```python
from build123d import *

# Parameters (mm, degrees)
CUT_EXTRUDE1_REACH             = 24.669
SKETCH2_R                      = 0.9525
CUT_EXTRUDE1_DIRECTION_2_REACH = 24.669


with BuildPart() as part:
    # Sketch3 → Revolve1 (revolve)
    with BuildSketch(Plane(origin=(0, 0, 0), x_dir=(0, 0, -1), z_dir=(1, 0, 0)), mode=Mode.PRIVATE) as revolve1_sk:
        with BuildLine():
            Line((-4.7625, 7.1247), (-4.7625, 9.50595))
            ThreePointArc((-4.7625, 9.50595), (-0.2272742, 11.825581937), (3.112721606, 15.6718))
            Line((3.112721606, 15.6718), (4.7625, 14.7193))
            Line((4.7625, 14.7193), (2.305035487, 10.462846606))
            ThreePointArc((2.305035487, 10.462846606), (2.305035487, 9.824915535), (2.8575, 9.50595))
            Line((2.8575, 9.50595), (4.28625, 9.50595))
            Line((4.28625, 9.50595), (4.28625, 7.1247))
            Line((4.28625, 7.1247), (-4.7625, 7.1247))
        make_face()
    revolve(revolve1_sk.sketch.rotate(Axis((0, 0, 4.7625), (0, 0, -1)), 180), axis=Axis((0, 0, 4.7625), (0, 0, -1)))

    # Sketch2 → Cut-Extrude1 (cut, up to next)
    with BuildSketch(Plane(origin=(0, 0, 0), x_dir=(0, 0, -1), z_dir=(1, 0, 0)), mode=Mode.PRIVATE) as cut_extrude1_sk1:
        with Locations((4.7625, 0)):
            Circle(SKETCH2_R)
    cut_extrude1_tool1 = extrude(cut_extrude1_sk1.sketch, amount=-CUT_EXTRUDE1_REACH, mode=Mode.PRIVATE) & part.part
    add(cut_extrude1_tool1.solids().sort_by_distance((0, 0, -4.7625))[0], mode=Mode.SUBTRACT)

    # Sketch2 → Cut-Extrude1 direction 2 (cut, up to next)
    with BuildSketch(Plane(origin=(0, 0, 0), x_dir=(0, 0, -1), z_dir=(1, 0, 0)), mode=Mode.PRIVATE) as cut_extrude1_direction_2_sk1:
        with Locations((4.7625, 0)):
            Circle(SKETCH2_R)
    cut_extrude1_direction_2_tool1 = extrude(cut_extrude1_direction_2_sk1.sketch, amount=CUT_EXTRUDE1_DIRECTION_2_REACH, mode=Mode.PRIVATE) & part.part
    add(cut_extrude1_direction_2_tool1.solids().sort_by_distance((0, 0, -4.7625))[0], mode=Mode.SUBTRACT)


solid = part.part
```
Input: part model. Units: mm. Frame: model coordinates. A direction names the side the tool comes from. Round coordinates to 2 decimals unless told otherwise and drop trailing zeros. Order: outer loops, then holes, each group sorted by start corner. A loop starts at its lowest first (then second) coordinate and runs counter-clockwise, first axis right, second up. Notation, with made-up numbers: (67, 83.5) - (87, 83.5) arc R13 cw to (87, 93.5) - close; hole circle Ø9 at (34.5, 19). An arc over 180 degrees is marked (long way). Answer in a Markdown table with one row per item.
Item 1: Section query C-C (z = 1.75). Return the cut outline in (x, y), then the cut area to 3 significant figures.
Model answer:
| item | result |
|---|---|
| outline | circle Ø21.59 at (0, 0); hole circle Ø14.25 at (0, 0) |
| area | 207 mm² |
Item 2: Mould query, pull axis X, two halves, no side actions, for faces 3 (the conical face through (-3.205, -10.177, -2.424)), 4 (the flat face through (-6.4, 3.5, 4.762)). Classes: released by +X, released by -X, zero draft, split by the parting line, or undercut.
Model answer:
| item | result |
|---|---|
| face 3 | undercut |
| face 4 | zero draft |
Item 3: Section query B-B (y = 0). Return the cut outline in (x, z), then the cut area to 3 significant figures.
Model answer:
| item | result |
|---|---|
| outline | (-15.67, -3.11) - (-14.72, -4.76) - (-10.46, -2.31) arc R0.64 cw to (-9.51, -2.86) - (-9.51, -3.81) - (-7.12, -3.81) - (-7.12, 4.76) - (-9.51, 4.76) arc R13.38 cw to start; (7.12, -3.81) - (9.51, -3.81) - (9.51, -2.86) arc R0.64 cw to (10.46, -2.31) - (14.72, -4.76) - (15.67, -3.11) arc R13.38 cw to (9.51, 4.76) - (7.12, 4.76) - close |
| area | 80.0 mm² |
Item 4: Section query D-D (z = -0.25). Return the cut outline in (x, y).
Model answer:
| item | result |
|---|---|
| outline | circle Ø24.43 at (0, 0); hole circle Ø14.25 at (0, 0) |
Item 5: Line query: line 1 (X direction, y = 2, z = -2.75); line 2 (X direction, y = -3, z = -2.75); line 3 (Z direction, x = -6, y = -4). Output: solid intervals per line, ascending.
Model answer:
| item | result |
|---|---|
| line 1 | x = -14.95 to -11.05, -9.3 to -6.84, 6.84 to 9.3, 11.05 to 14.95 |
| line 2 | x = -14.78 to -10.83, -9.03 to -6.46, 6.46 to 9.03, 10.83 to 14.78 |
| line 3 | z = -4.29 to 4.76 |
Item 6: Section query A-A (x = 0). Return the cut outline in (y, z), then the cut area to 3 significant figures.
Model answer:
| item | result |
|---|---|
| outline | (-15.67, -3.11) - (-14.72, -4.76) - (-10.46, -2.31) arc R0.64 cw to (-9.51, -2.86) - (-9.51, -4.29) - (-7.12, -4.29) - (-7.12, 4.76) - (-9.51, 4.76) arc R13.38 cw to start; (7.12, -4.29) - (9.51, -4.29) - (9.51, -2.86) arc R0.64 cw to (10.46, -2.31) - (14.72, -4.76) - (15.67, -3.11) arc R13.38 cw to (9.51, 4.76) - (7.12, 4.76) - close |
| area | 82.3 mm² |
Item 7: Pin query (flat end, axial travel): pin 1 (4.5 mm diameter, centred on x = -4.5, y = 6.5, fed in from -Z); pin 2 (1.5 mm diameter, centred on y = 0.5, z = -1, fed in from -X); pin 3 (8 mm diameter, centred on x = -9.5, y = -7, fed in from +Z); pin 4 (5 mm diameter, centred on y = -1.5, z = 2.5, fed in from +X). Return the tip coordinate at first contact, or that it passes through.
Model answer:
| item | result |
|---|---|
| pin 1 | stops at z = -4.29 |
| pin 2 | stops at x = -13.72 |
| pin 3 | stops at z = 4.76 |
| pin 4 | stops at x = 11.93 |
Item 8: Reachability of faces 1 (the flat face through (2, 7, -4.286)), 2 (the cylindrical face through (-4.815, 5.251, 0.301)) from +Z, -Z, +X, -X, +Y, -Y: full face, straight path, thin tool, end or side. Return the list, or none.
Model answer:
| item | result |
|---|---|
| face 1 | -Z |
| face 2 | +Z, -Z |
